Check sheet for the modelled part. Datum: model origin and axes. Units: mm. A direction names the side the tool comes from. Give positions to 0.01 mm unless a question says otherwise; leave off trailing zeros. Loops run counter-clockwise (first coordinate to the right, second up) from the corner with the lowest first, then second, coordinate; pieces in that order, holes last.
```python
from build123d import *

# Parameters (mm, degrees)
SKETCH3_R                       = 4.7625
OXIDIZER_INLET_HOLE_DEPTH       = 88.798079296
FLANGE_HOLES_D                  = 2.8702
DOWEL_HOLES_D                   = 4.7625
DOWEL_HOLES_DEPTH               = 6.35
DOWEL_HOLES_TIP                 = 1.430799349
SKETCH12_R                      = 38.1
IMPINGING_PLATE_FLAT_CUT_DEPTH  = 3.81
SKETCH14_R                      = 38.1
SKETCH15_R                      = 38.1
SKETCH16_R                      = 28.575
SKETCH17_R                      = 4.7625
INTERNAL_FILLET_R               = 3.175
EXTENDED_8_BC_COUNT             = 8
CHAMFER_FOR_IMPINGING_EDGE_SIZE = 0.127


with BuildPart() as part:
    # Sketch2 → Main Structure (revolve)
    with BuildSketch(Plane.XY, mode=Mode.PRIVATE) as main_structure_sk:
        Polygon((0, 0), (0, 56.35625), (9.525, 56.35625), (9.525, 45.72), (22.225, 13.081), (34.925, 13.081), (34.925, 6.2484), (36.83, 6.2484), (36.83, 0), align=None)
    revolve(main_structure_sk.sketch.rotate(Axis((0, 0, 0), (1, 0, 0)), 90), axis=Axis((0, 0, 0), (1, 0, 0)))

    # Sketch3 → Oxidizer Inlet Hole (cut, through all)
    with BuildSketch(Plane(origin=(36.83, 0, 0), x_dir=(0, 0, -1), z_dir=(1, 0, 0))):
        Circle(SKETCH3_R)
    extrude(amount=-OXIDIZER_INLET_HOLE_DEPTH, mode=Mode.SUBTRACT)

    # Flange Holes (through all)
    with Locations(Plane.ZY):
        with Locations((0, -51.6255), (-25.81275, -44.708994483), (-44.708994483, -25.81275), (-51.6255, 0), (-44.708994483, 25.81275), (-25.81275, 44.708994483), (0, 51.6255), (25.81275, 44.708994483), (44.708994483, 25.81275), (51.6255, 0), (44.708994483, -25.81275), (25.81275, -44.708994483)):
            Hole(FLANGE_HOLES_D / 2)

    # Dowel Holes
    with Locations(Plane.ZY):
        with Locations((49.866403745, -13.361662613), (-49.866403745, 13.361662613)):
            Hole(DOWEL_HOLES_D / 2, depth=DOWEL_HOLES_DEPTH)
            with Locations((0, 0, -(DOWEL_HOLES_DEPTH + DOWEL_HOLES_TIP / 2))):  # 118° drill point
                Cone(0, DOWEL_HOLES_D / 2, DOWEL_HOLES_TIP, mode=Mode.SUBTRACT)

    # Sketch12 → Impinging Plate Flat Cut (cut)
    with BuildSketch(Plane.ZY):
        Circle(SKETCH12_R)
    extrude(amount=-IMPINGING_PLATE_FLAT_CUT_DEPTH, mode=Mode.SUBTRACT)

    # Sketch14 → Impinging Plate Taper Cut section 0
    with BuildSketch(Plane.ZY.offset(-3.81)):
        Circle(SKETCH14_R)
    # Sketch15 → Impinging Plate Taper Cut section 1
    with BuildSketch(Plane.ZY.offset(-6.35)):
        Circle(SKETCH15_R)
    loft(mode=Mode.SUBTRACT)

    # Sketch16 → Internal Flow Path Loft Cut section 0
    with BuildSketch(Plane.ZY.offset(-6.35)):
        Circle(SKETCH16_R)
    # Sketch17 → Internal Flow Path Loft Cut section 1
    with BuildSketch(Plane.ZY.offset(-21.59)):
        Circle(SKETCH17_R)
    loft(mode=Mode.SUBTRACT)

    # Internal Fillet
    internal_fillet_edges = [part.edges().sort_by_distance(p)[0] for p in [
        (21.59, 4.7625, 0),
    ]]
    fillet(internal_fillet_edges, radius=INTERNAL_FILLET_R)

    # Sketch20 → 4-40 Tapped Holes (revolve, cut)
    with BuildSketch(Plane(origin=(6.35, 0, 33.3375), x_dir=(0, 0, 1), z_dir=(0, 1, 0))):
        Polygon((0, 0), (0, 3.854152758), (1.1303, 3.175), (1.1303, 0), align=None)
    f_4_40_tapped_holes = revolve(axis=Axis((0, 0, 33.3375), (1, 0, 0)), mode=Mode.SUBTRACT)

    # Extended 8 BC: 4-40 Tapped Holes ×8 about axis
    extended_8_bc_axis = Axis((0, 0, 0), (1, 0, 0))
    for i in range(1, EXTENDED_8_BC_COUNT):
        add(f_4_40_tapped_holes.rotate(extended_8_bc_axis, i * 360 / EXTENDED_8_BC_COUNT), mode=Mode.SUBTRACT)

    # Chamfer for Impinging Edge
    chamfer_for_impinging_edge_edges = [part.edges().sort_by_distance(p)[0] for p in [
        (6.35, 0, -38.1),
    ]]
    chamfer(chamfer_for_impinging_edge_edges, length=CHAMFER_FOR_IMPINGING_EDGE_SIZE)


solid = part.part
```
(1) Access from +Z, -Z, +X, -X, +Y, -Y to the whole of each face (thin tool, end or side, straight path). Record for faces 1 (the face through (3.22, -11.35, 48.59)), 2 (the face through (4.829, 25.263, -46.035)).
(2) Release check for a two-part mould opening along Y. For faces 3 (the face through (4.829, 43.436, 25.151)), 4 (the face through (9.525, 46, 8)), 5 (the face through (4.829, 34.292, -44.722)) record: pulls with the +Y half, pulls with the -Y half, needs draft (parallel to the pull), parting line crosses it, or undercut.
(3) Section check A-A on x = 29. Record the boundary of the cut face in (y, z) (1 decimal), plus the area to 3 significant figures.
(4) Section check B-B on x = 18.5. Record the boundary of the cut face in (y, z), plus the area to 3 significant figures.
(5) Material ranges on line 1 (Y direction, x = 3, z = 0); line 2 (Z direction, x = 9, y = -25); line 3 (Z direction, x = 6.5, y = -14.5), recorded low to high.
(6) Gauge pin test, flat ends, axial feed: pin 1 Ø2 at (y, z) = (-13, 22) entering from +X; pin 2 Ø2 at (y, z) = (23.57, 23.57) entering from +X; pin 3 Ø3.5 at (y, z) = (0, -33.34) entering from -X. Record the tip position at first contact, or that the pin passes through.
Computed values:
1. face 1: -X
1. face 2: +X, -X
2. face 3: undercut
2. face 4: needs draft
2. face 5: parting line crosses it
3. outline: circle Ø26.2 at (0, 0); hole circle Ø9.5 at (0, 0)
3. area: 466 mm2
4. outline: circle Ø45.31 at (0, 0); hole circle Ø19.18 at (0, 0)
4. area: 1,320 mm2
5. line 1: y = -56.36 to -53.06, -50.19 to -38.1, 38.1 to 50.19, 53.06 to 56.36
5. line 2: z = -50.51 to -45.89, -43.53 to 43.53, 45.89 to 50.51
5. line 3: z = -54.46 to -24.35, 24.35 to 48.06, 51.67 to 54.46
6. pin 1: stops at x = 17.76
6. pin 2: stops at x = 14.73
6. pin 3: stops at x = 6.35
